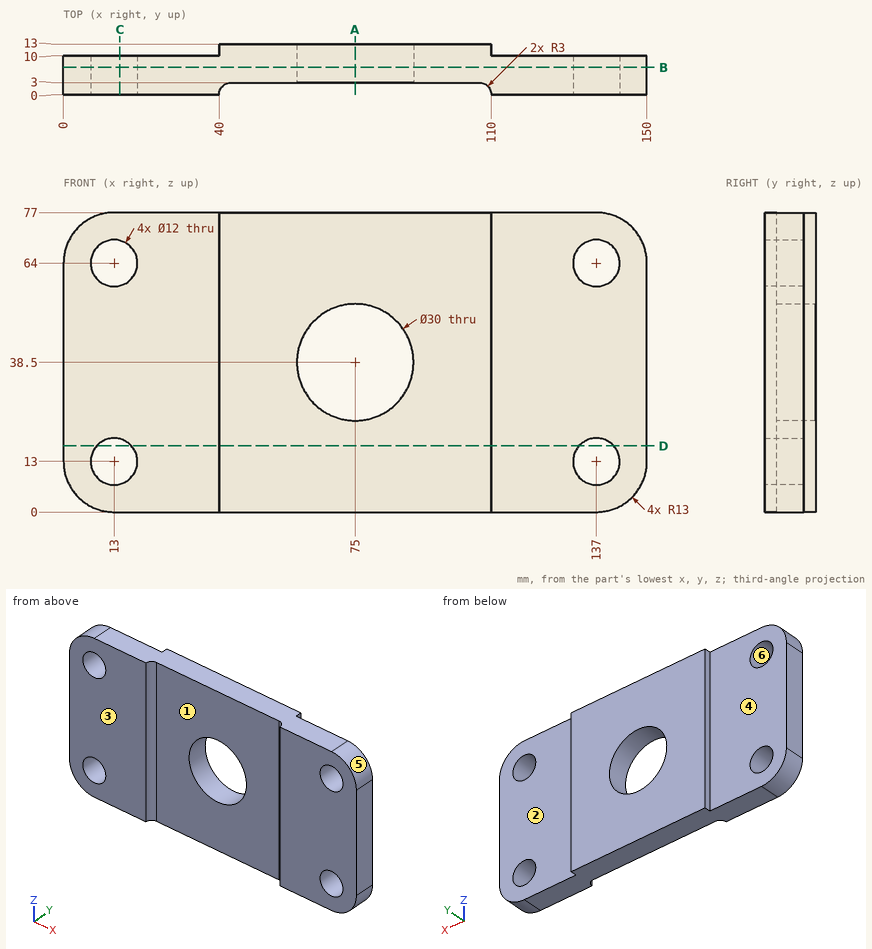
Can you work these out from the drawing? Everything is in mm from the part's minimum corner. A direction names the side the tool comes from. Coordinates: 2 decimals unless noted, no trailing zeros. Write each loop counter-clockwise with the first axis right and the second up, starting at its lowest first coordinate (ties: lowest second). Pieces come first, ordered by that corner, then holes. Notation, with made-up numbers: (78, 77.25) -> (85, 77.25) arc R30 ccw to (85, 108.25) -> close; hole circle Ø5 at (59, 26). An arc over 180 degrees is marked (long way). Return JSON: item names as keys, results as strings.
(1) Which directions (+Z, -Z, +X, -X, +Y, -Y) give clear straight access to the entire face, cutting with the end or side of a thin tool? Please do the marked faces 1, 2 and 3.
Numbers:
{"face 1": "+Z, -Z, -Y", "face 2": "+Z, -Z, +X, +Y", "face 3": "+Z, -Z, +X, -X, -Y"}
(2) Imagine slicing it at A-A, the plane x = 75. Please give me the cut outline in (y, z).
Numbers:
{"outline": "(3, 0) -> (13, 0) -> (13, 23.5) -> (3, 23.5) -> close; (3, 53.5) -> (13, 53.5) -> (13, 77) -> (3, 77) -> close"}
(3) We'd pull the mould along Z, two halves only. Please class the marked faces 4, 5 and 6: +Z half, -Z half, draft (parallel to the pull), parting line (faces both ways), or undercut.
Numbers:
{"face 4": "draft", "face 5": "+Z half", "face 6": "undercut"}
(4) I need wall thicknesses on L1, parallel to Z at x = 13, y = 3.5; L2, parallel to X at y = 4, z = 64; L3, parallel to X at y = 2.75, z = 64. Which ranges of each line are inside material? Lowest first, please.
Numbers:
{"L1": "z = 0 to 7, 19 to 58, 70 to 77", "L2": "x = 0 to 7, 19 to 131, 143 to 150", "L3": "x = 0 to 7, 19 to 41.8, 108.2 to 131, 143 to 150"}
(5) Imagine slicing it at C-C, the plane x = 14.5. Please give me the cut outline in (y, z), then the cut area to 3 significant figures.
Numbers:
{"outline": "(0, 0) -> (10, 0) -> (10, 7.19) -> (0, 7.19) -> close; (0, 18.81) -> (10, 18.81) -> (10, 58.19) -> (0, 58.19) -> close; (0, 69.81) -> (10, 69.81) -> (10, 77) -> (0, 77) -> close", "area": "538 mm2"}
(6) Imagine slicing it at B-B, the plane y = 7. Please give me the cut outline in (x, z), then the cut area to 3 significant figures.
Numbers:
{"outline": "(0, 13) arc R13 ccw to (13, 0) -> (137, 0) arc R13 ccw to (150, 13) -> (150, 64) arc R13 ccw to (137, 77) -> (13, 77) arc R13 ccw to (0, 64) -> close; hole circle Ø12 at (13, 13); hole circle Ø12 at (13, 64); hole circle Ø30 at (75, 38.5); hole circle Ø12 at (137, 13); hole circle Ø12 at (137, 64)", "area": "10,200 mm2"}
(7) I'm going to push flat-ended pins straight in: pin 1 (2.5 mm diameter, centred on y = 12, z = 47.5, fed in from -X); pin 2 (8 mm diameter, centred on x = 103, z = 9.5, fed in from -Y); pin 3 (2 mm diameter, centred on y = 11.5, z = 17.5, fed in from +X); pin 4 (9.5 mm diameter, centred on x = 13, z = 13, fed in from -Y). Where does each tip first touch, or does it pass through?
Numbers:
{"pin 1": "stops at x = 40", "pin 2": "stops at y = 3", "pin 3": "stops at x = 110", "pin 4": "passes through"}
(8) Imagine slicing it at D-D, the plane z = 17. Count the separate pieces of the cut face and the enclosed holes in it, then the cut area to 4 significant figures.
Numbers:
{"separate pieces": "3", "enclosed holes": "0", "area": "1,325 mm2"}
